Check sheet for the modelled part. Datum: model origin and axes. Units: mm. Face numbers are marked on the shaded views. A direction names the side the tool comes from. Round coordinates to 2 decimals unless told otherwise and drop trailing zeros. Loops run counter-clockwise (first coordinate to the right, second up) from the corner with the lowest first, then second, coordinate; pieces in that order, holes last. Notation, with made-up numbers: (-16.75, 13.25) - (4.25, 13.25) arc R3 cw to (4.25, 17.25) - close; hole circle Ø3 at (5.5, -3.75). An arc over 180 degrees is marked (long way). Answer in a Markdown table with one row per item. Add a question column.
(1) Access from +Z, -Z, +X, -X, +Y, -Y to the whole of each face (thin tool, end or side, straight path). Record for the marked faces 1, 2 and 3.
(2) Thickness scan on line 1 along Z through (x, y) = (0.5, 0.75); line 2 along Z through (x, y) = (-1.25, 5.25); line 3 along X through (y, z) = (4, -2.75). Record the ranges inside material, lowest first.
(3) Cross-section at B-B on z = 2.5. Enter the section's corners in (x, y).
(4) Mould release check, pull along X, two halves, no side actions. Record for the marked faces 4, 5, 6 and 7: +X half, -X half, draft (parallel to the pull), parting line (faces both ways), or undercut.
(5) Gauge pin test, flat ends, axial feed: pin 1 (1.5 mm diameter, centred on x = 0, y = 1.5, fed in from -Z); pin 2 (1.5 mm diameter, centred on y = 1, z = -3.5, fed in from -X); pin 3 (3 mm diameter, centred on y = 4.5, z = -4, fed in from +X). Record the tip position at first contact, or that the pin passes through.
(6) Cross-section at A-A on x = -2. Enter the section's corners in (y, z), then the cut area to 3 significant figures.
(7) Cross-section at C-C on x = 9.25. Count the separate pieces of the cut face and the enclosed holes in it, then the cut area to 3 significant figures.
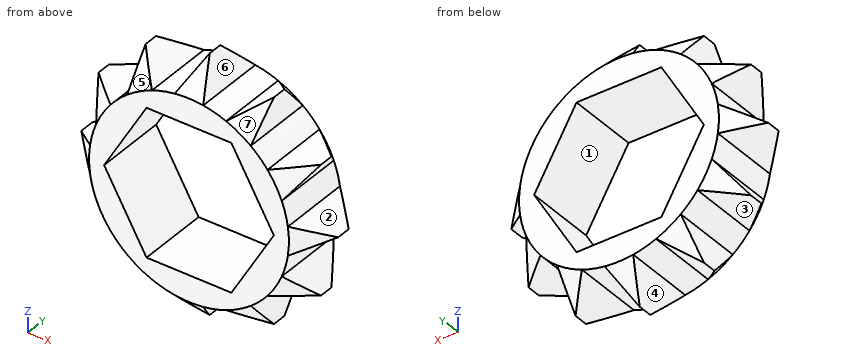
from build123d import *

# Parameters (mm, degrees)
SKETCH1_R           = 8.89
BOSS_EXTRUDE1_DEPTH = 6.35


with BuildPart() as part:
    # Sketch1 → Boss-Extrude1 (new body)
    # profile 1 of 13: a face of its own
    with BuildSketch(Plane(origin=(0, 0, 0), x_dir=(1, 0, 0), z_dir=(0, 1, 0))):
        Circle(SKETCH1_R)
        Polygon((3.776159436, -6.5405), (7.552318871, 0), (3.776159436, 6.5405), (-3.776159436, 6.5405), (-7.552318871, 0), (-3.776159436, -6.5405), align=None, mode=Mode.SUBTRACT)
    # profile 2 of 13: a face of its own
    with BuildSketch(Plane(origin=(0, 0, 0), x_dir=(1, 0, 0), z_dir=(0, 1, 0))):
        with BuildLine():
            ThreePointArc((-8.798818102, -1.27), (-8.89, 0), (-8.798818102, 1.27))
            Line((-8.798818102, 1.27), (-11.43, 0))
            Line((-11.43, 0), (-8.798818102, -1.27))
        make_face()
    # profile 3 of 13: a face of its own
    with BuildSketch(Plane(origin=(0, 0, 0), x_dir=(1, 0, 0), z_dir=(0, 1, 0))):
        with BuildLine():
            ThreePointArc((-6.985, -5.499261314), (-7.69896584, -4.445), (-8.255, -3.299556788))
            Line((-8.255, -3.299556788), (-9.898670365, -5.715))
            Line((-9.898670365, -5.715), (-6.985, -5.499261314))
        make_face()
    # profile 4 of 13: a face of its own
    with BuildSketch(Plane(origin=(0, 0, 0), x_dir=(1, 0, 0), z_dir=(0, 1, 0))):
        with BuildLine():
            ThreePointArc((-3.299556788, -8.255), (-4.445, -7.69896584), (-5.499261314, -6.985))
            Line((-5.499261314, -6.985), (-5.715, -9.898670365))
            Line((-5.715, -9.898670365), (-3.299556788, -8.255))
        make_face()
    # profile 5 of 13: a face of its own
    with BuildSketch(Plane(origin=(0, 0, 0), x_dir=(1, 0, 0), z_dir=(0, 1, 0))):
        with BuildLine():
            ThreePointArc((1.27, -8.798818102), (0, -8.89), (-1.27, -8.798818102))
            Line((-1.27, -8.798818102), (0, -11.43))
            Line((0, -11.43), (1.27, -8.798818102))
        make_face()
    # profile 6 of 13: a face of its own
    with BuildSketch(Plane(origin=(0, 0, 0), x_dir=(1, 0, 0), z_dir=(0, 1, 0))):
        with BuildLine():
            Line((5.715, -9.898670365), (5.499261314, -6.985))
            ThreePointArc((5.499261314, -6.985), (4.445, -7.69896584), (3.299556788, -8.255))
            Line((3.299556788, -8.255), (5.715, -9.898670365))
        make_face()
    # profile 7 of 13: a face of its own
    with BuildSketch(Plane(origin=(0, 0, 0), x_dir=(1, 0, 0), z_dir=(0, 1, 0))):
        with BuildLine():
            Line((9.898670365, -5.715), (8.255, -3.299556788))
            ThreePointArc((8.255, -3.299556788), (7.69896584, -4.445), (6.985, -5.499261314))
            Line((6.985, -5.499261314), (9.898670365, -5.715))
        make_face()
    # profile 8 of 13: a face of its own
    with BuildSketch(Plane(origin=(0, 0, 0), x_dir=(1, 0, 0), z_dir=(0, 1, 0))):
        with BuildLine():
            Line((11.43, 0), (8.798818102, 1.27))
            ThreePointArc((8.798818102, 1.27), (8.867175225, 0.636634538), (8.89, 0))
            ThreePointArc((8.89, 0), (8.867175225, -0.636634538), (8.798818102, -1.27))
            Line((8.798818102, -1.27), (11.43, 0))
        make_face()
    # profile 9 of 13: a face of its own
    with BuildSketch(Plane(origin=(0, 0, 0), x_dir=(1, 0, 0), z_dir=(0, 1, 0))):
        with BuildLine():
            Line((9.898670365, 5.715), (6.985, 5.499261314))
            ThreePointArc((6.985, 5.499261314), (7.69896584, 4.445), (8.255, 3.299556788))
            Line((8.255, 3.299556788), (9.898670365, 5.715))
        make_face()
    # profile 10 of 13: a face of its own
    with BuildSketch(Plane(origin=(0, 0, 0), x_dir=(1, 0, 0), z_dir=(0, 1, 0))):
        with BuildLine():
            Line((5.715, 9.898670365), (3.299556788, 8.255))
            ThreePointArc((3.299556788, 8.255), (4.445, 7.69896584), (5.499261314, 6.985))
            Line((5.499261314, 6.985), (5.715, 9.898670365))
        make_face()
    # profile 11 of 13: a face of its own
    with BuildSketch(Plane(origin=(0, 0, 0), x_dir=(1, 0, 0), z_dir=(0, 1, 0))):
        with BuildLine():
            Line((1.27, 8.798818102), (0, 11.43))
            Line((0, 11.43), (-1.27, 8.798818102))
            ThreePointArc((-1.27, 8.798818102), (0, 8.89), (1.27, 8.798818102))
        make_face()
    # profile 12 of 13: a face of its own
    with BuildSketch(Plane(origin=(0, 0, 0), x_dir=(1, 0, 0), z_dir=(0, 1, 0))):
        with BuildLine():
            ThreePointArc((-5.499261314, 6.985), (-4.445, 7.69896584), (-3.299556788, 8.255))
            Line((-3.299556788, 8.255), (-5.715, 9.898670365))
            Line((-5.715, 9.898670365), (-5.499261314, 6.985))
        make_face()
    # profile 13 of 13: a face of its own
    with BuildSketch(Plane(origin=(0, 0, 0), x_dir=(1, 0, 0), z_dir=(0, 1, 0))):
        with BuildLine():
            ThreePointArc((-8.255, 3.299556788), (-7.69896584, 4.445), (-6.985, 5.499261314))
            Line((-6.985, 5.499261314), (-9.898670365, 5.715))
            Line((-9.898670365, 5.715), (-8.255, 3.299556788))
        make_face()
    extrude(amount=BOSS_EXTRUDE1_DEPTH)

    # Sketch2 → Cut-Revolve1 (revolve, cut)
    with BuildSketch(Plane.XY):
        Polygon((-11.43, 3.81), (-8.89, 6.35), (-11.43, 6.35), align=None)
        Polygon((-11.43, 0), (-8.89, 0), (-11.43, 2.54), align=None)
    revolve(axis=Axis((0, 0, 0), (0, 1, 0)), mode=Mode.SUBTRACT)


solid = part.part
Answers:
| question | item | result |
|---|---|---|
| 1 | face 1 | +Y, -Y |
| 1 | face 2 | +X, +Y, -Y |
| 1 | face 3 | -Z, +Y, -Y |
| 2 | line 1 | z = -9.63 to -6.54, 6.54 to 9.63 |
| 2 | line 2 | z = -8.84 to -6.54, 6.54 to 8.84 |
| 2 | line 3 | x = -8.45 to -5.96, 5.96 to 8.45 |
| 3 | outline | (-8.53, 0) - (-6.11, 0) - (-6.11, 6.35) - (-8.53, 6.35) - close; (6.11, 0) - (8.53, 0) - (8.53, 6.35) - (6.11, 6.35) - close |
| 4 | face 4 | undercut |
| 4 | face 5 | -X half |
| 4 | face 6 | undercut |
| 4 | face 7 | +X half |
| 5 | pin 1 | stops at z = -11.14 |
| 5 | pin 2 | stops at x = -8.9 |
| 5 | pin 3 | stops at x = 9.72 |
| 6 | outline | (0, -8.66) - (6.35, -8.66) - (6.35, -6.54) - (0, -6.54) - close; (0, 6.54) - (6.35, 6.54) - (6.35, 8.66) - (0, 8.66) - close |
| 6 | area | 26.9 mm^2 |
| 7 | separate pieces | 3 |
| 7 | enclosed holes | 0 |
| 7 | area | 17.0 mm^2 |
